```python
from build123d import *

# Parameters (mm, degrees)
F1_DEPTH = 0.55
F2_W     = 4.5
F2_H     = 2.5
F3_DEPTH = 1.95
F4_R     = 1.24999
F5_R     = 0.7
F6_DEPTH = 25


# Not quite as in the source:
# - a fillet or chamfer is up to 0.001 mm smaller than in the source, because OpenCascade refuses the exact size


with BuildPart() as f1:
    # F0 (on Top) → F1 (new body)
    with BuildSketch(Plane.XY):
        with BuildLine():
            Line((7.1757397782, 1.55), (12, 1.55))
            Line((12, 1.55), (12, 4.05))
            Line((12, 4.05), (7.1757397782, 4.05))
            ThreePointArc((7.1757397782, 4.05), (6.8353451552, 4.0707678217), (6.5, 4.1327632138))
            ThreePointArc((6.5, 4.1327632138), (6.1928359056, 4.2281876541), (5.8986420809, 4.3582091838))
            Line((5.8986420809, 4.3582091838), (4.0770976972, 5.2917908162))
            ThreePointArc((4.0770976972, 5.2917908162), (3.4568811592, 5.5218572965), (2.8, 5.6))
            Line((2.8, 5.6), (2.8, 4.4))
            ThreePointArc((2.8, 4.4), (3.9313708499, 3.9313708499), (4.4, 2.8))
            ThreePointArc((4.4, 2.8), (3.9313708499, 1.6686291501), (2.8, 1.2))
            Line((2.8, 1.2), (2.8, 0))
            ThreePointArc((2.8, 0), (3.4568811592, 0.0781427035), (4.0770976972, 0.3082091838))
            Line((4.0770976972, 0.3082091838), (5.8986420809, 1.2417908162))
            ThreePointArc((5.8986420809, 1.2417908162), (6.1928359056, 1.3718123459), (6.5, 1.4672367862))
            ThreePointArc((6.5, 1.4672367862), (6.8353451552, 1.5292321783), (7.1757397782, 1.55))
        make_face()
        with BuildLine():
            ThreePointArc((0, 2.8), (0.8201010127, 0.8201010127), (2.8, 0))
            Line((2.8, 0), (2.8, 1.2))
            ThreePointArc((2.8, 1.2), (1.2, 2.8), (2.8, 4.4))
            Line((2.8, 4.4), (2.8, 5.6))
            ThreePointArc((2.8, 5.6), (0.8201010127, 4.7798989873), (0, 2.8))
        make_face()
    extrude(amount=F1_DEPTH)

    # F2 (on face) → F3 (join)
    with BuildSketch(Plane.XY.offset(0.55)):
        with Locations((9.75, 2.8)):
            Rectangle(F2_W, F2_H)
    extrude(amount=F3_DEPTH)

    # F4 (radius 1.25 in the source; OpenCascade refuses exactly that, so slightly less here)
    f4_edges = [f1.edges().sort_by_distance(p)[0] for p in [
        (9.75, 1.55, 2.5),
        (9.75, 4.05, 2.5),
    ]]
    fillet(f4_edges, radius=F4_R)

    # F5 (on face) → F6 (cut)
    with BuildSketch(Plane.YZ.offset(12)):
        with Locations((2.8, 1.25)):
            Circle(F5_R)
    extrude(amount=-F6_DEPTH, mode=Mode.SUBTRACT)


solid = f1.part
```
Model file for the job. Use its own axes, mm. A direction names the side the tool comes from. Round coordinates to 2 decimals unless told otherwise and drop trailing zeros. Order: outer loops, then holes, each group sorted by start corner. A loop starts at its lowest first (then second) coordinate and runs counter-clockwise, first axis right, second up. Notation, with made-up numbers: M -2.5,48 L 49.5,48 A29 ccw 49.5,69 Z; hole C 71,-19.5 d9. An arc over 180 degrees is marked long. Use CSV: the item, a comma, the result in double quotes.
Item 1: Probe probe 1 along Y at (x, z) = (10.05, 1.25); probe 2 along Z at (x, y) = (8.55, 2.8). List the from-to ranges inside material, lowest first.
Worked answers:
probe 1,"1.55 to 2.1, 3.5 to 4.05"
probe 2,"0 to 0.55, 1.95 to 2.5"
Item 2: Pull direction Z, two halves, no side cores. Call faces 4 (the face through (10, 4.05, 1)), 5 (the face through (9.782, 3.123, 0.629)), 6 (the face through (9.782, 1.926, 2.144)): released by +Z, released by -Z, zero draft, split by the parting line, or undercut.
Worked answers:
face 4,"zero draft"
face 5,"undercut"
face 6,"released by +Z"
Item 3: Saw through at D-D (z = 0.4). List the corners of the cut face in (x, y).
Worked answers:
outline,"M 4.08,0.31 L 5.9,1.24 A2.8 cw 7.18,1.55 L 12,1.55 L 12,4.05 L 7.18,4.05 A2.8 cw 5.9,4.36 L 4.08,5.29 A2.8 ccw long Z; hole C 2.8,2.8 d3.2"
Item 4: Saw through at C-C (x = 3.75). List the corners of the cut face in (y, z), plus the area to 3 significant figures.
Worked answers:
outline,"M 0.17,0 L 1.51,0 L 1.51,0.55 L 0.17,0.55 Z; M 4.09,0 L 5.43,0 L 5.43,0.55 L 4.09,0.55 Z"
area,"1.48 mm²"
Item 5: Which spindle directions (+Z, -Z, +X, -X, +Y, -Y) get a long thin tool onto all of the face, cutting with end or side? Do faces 1 (the face through (10, 1.55, 1)), 2 (the face through (7.5, 2, 2)), 3 (the face through (12, 2.8, 0.4)). Say none if no direction does.
Worked answers:
face 1,"+Z, -Z, +X, -Y"
face 2,"+Z, -X, +Y, -Y"
face 3,"+Z, -Z, +X, +Y, -Y"
Item 6: Saw through at B-B (z = 1.75). List the corners of the cut face in (x, y).
Worked answers:
outline,"M 7.5,1.65 L 12,1.65 L 12,2.31 L 7.5,2.31 Z; M 7.5,3.29 L 12,3.29 L 12,3.95 L 7.5,3.95 Z"
